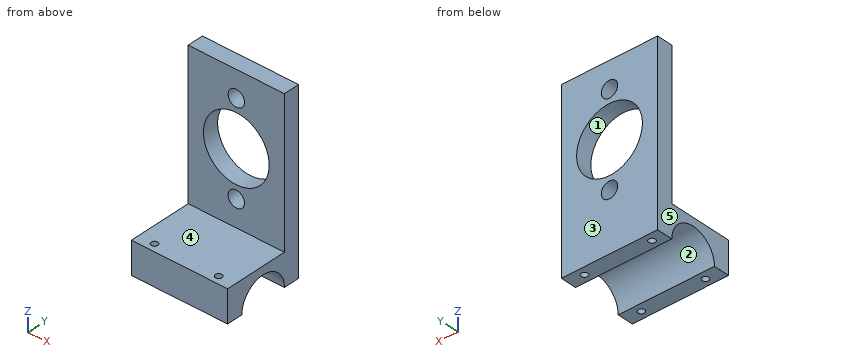
Solid Edge part; units mm, degrees
sketch "Sketch1" plane through (0, 0, 0) normal (0, -1, 0) x (1, 0, 0)
  line L0 (60.0075, 0) -> (60.0075, 110)
  line L1 (60.0075, 110) -> (0, 110)
  line L2 (0, 110) -> (0, 0)
  line L3 (0, 0) -> (60.0075, 0)
  circle A0 centre (30.0038, 93.6) radius 5.1
  circle A1 centre (30.0037, 36.4) radius 5.1
  circle A2 centre (30.0037, 65) radius 20.5
extrude "Protrusion1" add sketch "Sketch1" along normal blind 10
sketch "Sketch2" plane through (0, 0, 0) normal (0, -1, 0) x (1, 0, 0)
  line L0 (0, 20) -> (60.0075, 20)
  line L1 (60.0075, 20) -> (60.0075, 0)
  line L2 (60.0075, 0) -> (0, 0)
  line L3 (0, 0) -> (0, 20)
extrude "övre_fäste_protrusion" add sketch "Sketch2" along normal blind 50
sketch "Sketch3" plane through (60.0075, -20, 55) normal (1, 0, 0) x (0, 1, 0)
  circle A0 centre (-5, -55) radius 15
extrude "Halvcirkel_cutout" cut sketch "Sketch3" against normal blind 100
hole "Hole_1" at (10, -45, 0) direction (0, 0, 1) diameter 4.134 depth 20
hole "Hole1" at (50.0075, -45, 0) direction (0, 0, 1) diameter 4.134 depth 20
hole "Hole2" at (7.933, -5, 0) direction (0, 0, 1) diameter 4.134 depth 20
hole "Hole3" at (50.0075, -5, 0) direction (0, 0, 1) diameter 4.134 depth 20
CAD build for the part. Positions are in the model's coordinates, mm. Face numbers are marked on the shaded views. A direction names the side the tool comes from. Coordinates: 2 decimals unless noted, no trailing zeros. Write each loop counter-clockwise with the first axis right and the second up, starting at its lowest first coordinate (ties: lowest second). Pieces come first, ordered by that corner, then holes.
(1) 3-axis set-ups, long thin cutter, end or side, ignore diameter. For the marked faces 4 and 5: which of +Z, -Z, +X, -X, +Y, -Y reach the whole face in a straight line?
(2) Two-plate mould, pull along Y, no slides. Class the marked faces 1, 2 and 3: +Y half, -Y half, draft (parallel to the pull), parting line (faces both ways), or undercut.
(3) Drill centre lines: probe 1 along X at (y, z) = (-45, 11.75); probe 2 along Y at (x, z) = (16.5, 24); probe 3 along Z at (x, y) = (57.5, -25.5). Where is each one in solid material? Low to high.
(4) Flat gauge pins, fed straight in: pin 1 (1.5 mm diameter, centred on x = 53.5, y = -31, fed in from +Z); pin 2 (1.5 mm diameter, centred on x = 26.5, y = -23, fed in from -Z). Where does each tip first touch, or does it go through?
(5) Cut at A-A, the plane z = 65. List the corners of the cut face in (x, y).
(6) Cut at D-D, the plane y = -5. List the corners of the cut face in (x, z).
(7) Cut at C-C, the plane x = 32.5. List the corners of the cut face in (y, z).
(8) Cut at B-B, the plane y = -45. List the corners of the cut face in (x, z).
Geometry says:
1. face 4: +Z, +X, -X, -Y
1. face 5: +Z, -Z, -X, +Y, -Y
2. face 1: draft
2. face 2: undercut
2. face 3: +Y half
3. probe 1: x = 0 to 7.93, 12.07 to 47.94, 52.07 to 60.01
3. probe 2: y = -10 to 0
3. probe 3: z = 14.99 to 20
4. pin 1: stops at z = 20
4. pin 2: stops at z = 14.75
5. outline: (0, -10) - (9.5, -10) - (9.5, 0) - (0, 0) - close; (50.5, -10) - (60.01, -10) - (60.01, 0) - (50.5, 0) - close
6. outline: (0, 0) - (5.87, 0) - (5.87, 20) - (10, 20) - (10, 0) - (47.94, 0) - (47.94, 20) - (52.07, 20) - (52.07, 0) - (60.01, 0) - (60.01, 110) - (0, 110) - close; hole circle Ø41 at (30, 65); hole circle Ø10.2 at (30, 36.4); hole circle Ø10.2 at (30, 93.6)
7. outline: (-50, 0) - (-40, 0) arc R15 cw to (-10, 0) - (0, 0) - (0, 31.95) - (-10, 31.95) - (-10, 20) - (-50, 20) - close; (-10, 40.85) - (0, 40.85) - (0, 44.65) - (-10, 44.65) - close; (-10, 85.35) - (0, 85.35) - (0, 89.15) - (-10, 89.15) - close; (-10, 98.05) - (0, 98.05) - (0, 110) - (-10, 110) - close
8. outline: (0, 0) - (7.93, 0) - (7.93, 20) - (0, 20) - close; (12.07, 0) - (47.94, 0) - (47.94, 20) - (12.07, 20) - close; (52.07, 0) - (60.01, 0) - (60.01, 20) - (52.07, 20) - close
